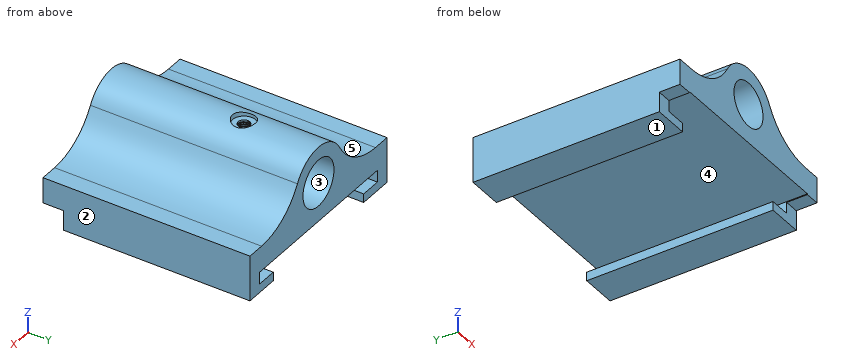
```python
from build123d import *

# Parameters (mm, degrees)
BOSS_EXTRUDE1_DEPTH = 50
SKETCH2_W           = 50
SKETCH2_H           = 4.8
CUT_EXTRUDE1_DEPTH  = 5
SKETCH3_R           = 5.3
CUT_EXTRUDE2_DEPTH  = 72.561162651
BOSS_EXTRUDE2_DEPTH = 50
FILLET1_R           = 15
SKETCH6_R           = 1.4
CUT_EXTRUDE4_DEPTH  = 10
SKETCH7_R           = 2.75
CUT_EXTRUDE5_DEPTH  = 5
THREAD1_PITCH       = 0.5
SKETCH9_R           = 5.65
CUT_EXTRUDE6_DEPTH  = 10


with BuildPart() as part:
    # Sketch1 → Boss-Extrude1 (new body)
    with BuildSketch(Plane(origin=(0, 0, 0), x_dir=(1, 0, 0), z_dir=(0, 1, 0))):
        Polygon((8.5, 0), (0, 0), (0, -11), (50, -11), (50, 0), (41.5, 0), (41.5, -2.104480912), (46.5, -2.104480912), (46.5, -5), (3.5, -5), (3.5, -2.104480912), (8.5, -2.104480912), align=None)
    extrude(amount=BOSS_EXTRUDE1_DEPTH)

    # Sketch2 → Cut-Extrude1 (cut)
    with BuildSketch(Plane.XZ):
        with Locations((25, 2.4)):
            Rectangle(SKETCH2_W, SKETCH2_H)
    extrude(amount=-CUT_EXTRUDE1_DEPTH, mode=Mode.SUBTRACT)

    # Sketch3 → Cut-Extrude2 (cut, through all)
    with BuildSketch(Plane(origin=(0, 50, 0), x_dir=(1, 0, 0), z_dir=(0, 1, 0))):
        with Locations((25, -14.412334908)):
            Circle(SKETCH3_R)
    extrude(amount=-CUT_EXTRUDE2_DEPTH, mode=Mode.SUBTRACT)

    # Sketch5 → Boss-Extrude2 (add)
    with BuildSketch(Plane(origin=(0, 50, 0), x_dir=(1, 0, 0), z_dir=(0, 1, 0))):
        with BuildLine():
            Line((16.888528464, -11), (20.944636826, -11))
            ThreePointArc((20.944636826, -11), (25, -19.712334908), (29.055363174, -11))
            Line((29.055363174, -11), (33.111471536, -11))
            ThreePointArc((33.111471536, -11), (25, -23.212334908), (16.888528464, -11))
        make_face()
    extrude(amount=-BOSS_EXTRUDE2_DEPTH)

    # Fillet1
    fillet1_edges = [part.edges().sort_by_distance(p)[0] for p in [
        (33.111471536, 25, 11),
        (16.888528464, 25, 11),
    ]]
    fillet(fillet1_edges, radius=FILLET1_R)

    # Sketch6 → Cut-Extrude4 (cut)
    with BuildSketch(Plane.XY.offset(27)):
        with Locations((25, 32)):
            Circle(SKETCH6_R)
    extrude(amount=-CUT_EXTRUDE4_DEPTH, mode=Mode.SUBTRACT)

    # Sketch7 → Cut-Extrude5 (cut)
    with BuildSketch(Plane.XY.offset(27)):
        with Locations((25, 32)):
            Circle(SKETCH7_R)
    extrude(amount=-CUT_EXTRUDE5_DEPTH, mode=Mode.SUBTRACT)

    # Thread1: the profile of Thread Profile1 profile screwed along a right-hand helix of 4.4 turns, 6 arcs to a turn; built about Z, then put on its axis
    thread1_z = Axis((0, 0, 0), (0, 0, 1))
    thread1_corners = [(1.4003, 0, -0.000173205), (1.4003, 0, 0.218923204), (1.264683531, 0, 0.140625), (1.264683531, 0, 0.078125)]
    with BuildLine(mode=Mode.PRIVATE) as thread1_profile:
        Line(thread1_corners[0], thread1_corners[1])
        Line(thread1_corners[1], thread1_corners[2])
        Line(thread1_corners[2], thread1_corners[3])
        Line(thread1_corners[3], thread1_corners[0])
    thread1_cap = Face(thread1_profile.wire())
    thread1_turn_angles = [0, 30, 60, 90, 120, 150, 180, 210, 240, 270, 300, 330, 360]
    thread1_turn_weights = [1, 0.8660254037844387, 1, 0.8660254037844387, 1, 0.8660254037844387, 1, 0.8660254037844387, 1, 0.8660254037844387, 1, 0.8660254037844387, 1]
    thread1_turn_rails = [Edge.make_bspline([Vector(p[0], p[1], 0).rotate(thread1_z, thread1_turn_angles[k]) / thread1_turn_weights[k] + Vector(0, 0, p[2] + THREAD1_PITCH * thread1_turn_angles[k] / 360) for k in range(13)], [0, 0, 0, 1, 1, 2, 2, 3, 3, 4, 4, 5, 5, 6, 6, 6], 2, thread1_turn_weights) for p in thread1_corners]
    thread1_turn_sides = [Face.make_surface_from_curves(thread1_turn_rails[p[0]], thread1_turn_rails[p[1]]) for p in [(0, 1), (1, 2), (2, 3), (3, 0)]]
    thread1_last_angles = [1440, 1470, 1500, 1530, 1560, 1572, 1584]
    thread1_last_weights = [1, 0.8660254037844387, 1, 0.8660254037844387, 1, 0.9781476007338052, 1]
    thread1_last_rails = [Edge.make_bspline([Vector(p[0], p[1], 0).rotate(thread1_z, thread1_last_angles[k]) / thread1_last_weights[k] + Vector(0, 0, p[2] + THREAD1_PITCH * thread1_last_angles[k] / 360) for k in range(7)], [0, 0, 0, 1, 1, 2, 2, 3, 3, 3], 2, thread1_last_weights) for p in thread1_corners]
    thread1_last_sides = [Face.make_surface_from_curves(thread1_last_rails[p[0]], thread1_last_rails[p[1]]) for p in [(0, 1), (1, 2), (2, 3), (3, 0)]]
    thread1 = Plane(origin=(25, 32, 22), x_dir=(-1, 0, 0), z_dir=(0, 0, -1)) * Solid(Shell([*[p.moved(Location((0, 0, THREAD1_PITCH * i))) for i in range(4) for p in thread1_turn_sides], *thread1_last_sides, thread1_cap, thread1_cap.rotate(thread1_z, 1584).moved(Location((0, 0, THREAD1_PITCH * 1584 / 360)))]))
    add(thread1)

    # Sketch9 → Cut-Extrude6 (cut)
    with BuildSketch(Plane(origin=(0, 50, 0), x_dir=(1, 0, 0), z_dir=(0, 1, 0))):
        with Locations(Location((25, -14.412334908, 0), (0, 0, 270))):
            Circle(SKETCH9_R)
    extrude(amount=-CUT_EXTRUDE6_DEPTH, mode=Mode.SUBTRACT)


solid = part.part
```
Geometry check sheet. Reference: the model listing, model coordinates, mm. Face numbers are marked on the shaded views. A direction names the side the tool comes from. Round coordinates to 2 decimals unless told otherwise and drop trailing zeros. Loops run counter-clockwise (first coordinate to the right, second up) from the corner with the lowest first, then second, coordinate; pieces in that order, holes last. Notation, with made-up numbers: M 89,-30 L 129,-30 A19 cw 129,5 Z; hole C 2.5,14.5 d9. An arc over 180 degrees is marked long. Return JSON: item names as keys, results as strings. Group by question number.
(1) Go/stop test with flat-tipped pins: pin 1 (2 mm diameter, centred on x = 3, y = 18, fed in from +Z); pin 2 (9 mm diameter, centred on x = 25, y = 32, fed in from -Z); pin 3 (10 mm diameter, centred on x = 38, y = 19, fed in from +Z). Record where each tip stops, or that it passes through.
(2) Section check A-A, the plane y = 37.5. Enter the section's corners in (x, z), and give its area (3 significant figures).
(3) Section check C-C, the plane x = 44. Enter the section's corners in (y, z), and give its area (3 significant figures).
(4) Mould release check, pull along Z, two halves, no side actions. Record for the marked faces 1, 2 and 3: pulls with the +Z half, pulls with the -Z half, needs draft (parallel to the pull), parting line crosses it, or undercut.
(5) Scan lines: line 1 along X through (y, z) = (11, 1.5); line 2 along X through (y, z) = (32, 3.5); line 3 along Y through (x, z) = (25, 22.3). Record each from-to range of solid material in increasing order. Write a range as [from, to].
(6) Section check D-D, the plane z = 17.25. Enter the section's corners in (x, y).
(7) Section check B-B, the plane z = 4. Enter the section's corners in (x, y), and give its area (3 significant figures).
(8) Set-up check for the marked faces 4 and 5: record each of +Z, -Z, +X, -X, +Y, -Y from which the full face is reachable in a straight line by a thin tool's end or side.
Data:
{
 "1": {"pin 1": "z = 11", "pin 2": "z = 5", "pin 3": "z = 18.16"},
 "2": {"outline": "M 0,0 L 8.5,0 L 8.5,2.1 L 3.5,2.1 L 3.5,5 L 46.5,5 L 46.5,2.1 L 41.5,2.1 L 41.5,0 L 50,0 L 50,11 L 45.79,11 A15 cw 32.69,18.7 A8.8 ccw 17.31,18.7 A15 cw 4.21,11 L 0,11 Z; hole C 25,14.41 d10.6", "area": "494 mm²"},
 "3": {"outline": "M 0,5 L 50,5 L 50,11.11 L 0,11.11 Z; M 5,0 L 50,0 L 50,2.1 L 5,2.1 Z", "area": "400 mm²"},
 "4": {"face 1": "pulls with the -Z half", "face 2": "needs draft", "face 3": "undercut"},
 "5": {"line 1": "[0, 8.5], [41.5, 50]", "line 2": "[0, 3.5], [46.5, 50]", "line 3": "[0, 29.25], [34.75, 50]"},
 "6": {"outline": "M 16.39,0 L 20.52,0 L 20.52,40 L 20.11,40 L 20.11,50 L 16.39,50 Z; M 29.48,0 L 33.61,0 L 33.61,50 L 29.89,50 L 29.89,40 L 29.48,40 Z"},
 "7": {"outline": "M 0,5 L 3.5,5 L 3.5,50 L 0,50 Z; M 46.5,5 L 50,5 L 50,50 L 46.5,50 Z", "area": "315 mm²"},
 "8": {"face 4": "+Y, -Y", "face 5": "+Z, -X, +Y, -Y"}
}
